For this review, take the finished solid that the model builds, in its own axes (mm). A direction names the side the tool comes from. Coordinates: 2 decimals unless noted, no trailing zeros. Write each loop counter-clockwise with the first axis right and the second up, starting at its lowest first coordinate (ties: lowest second). Pieces come first, ordered by that corner, then holes. Notation, with made-up numbers: M 4,16 L 63,16 A18 cw 63,31 Z; hole C 81,-31.75 d7. An arc over 180 degrees is marked long. Return JSON: item names as keys, results as strings.
```python
from build123d import *

# Parameters (mm, degrees)
F0_R     = 12.7
F1_DEPTH = 25.4
F2_R     = 6.35
F3_DEPTH = 12.7
F4_R     = 9.525
F5_DEPTH = 50.8


with BuildPart() as f1:
    # F0 (on Front) → F1 (new body)
    with BuildSketch(Plane.XZ):
        Circle(F0_R)
    extrude(amount=F1_DEPTH)

    # F2 (on face) → F3 (join)
    with BuildSketch(Plane(origin=(0, 0, 0), x_dir=(-1, 0, 0), z_dir=(0, 1, 0))):
        Circle(F2_R)
    extrude(amount=F3_DEPTH)

    # F4 (on face) → F5 (join)
    with BuildSketch(Plane.XZ.offset(25.4)):
        Circle(F4_R)
    extrude(amount=F5_DEPTH)


solid = f1.part
```
1. We need section D-D (y = -29). State the section outline as (x, z) points (3 decimals), plus the area to 3 significant figures.
Checks:
{"outline": "C 0,0 d19.05", "area": "285 mm2"}
2. Clearance check with flat-ended pins moving along their axes: pin 1 Ø6 at (x, y) = (4, -15) entering from +Z; pin 2 Ø6 at (x, y) = (6.5, -30) entering from -Z; pin 3 Ø4 at (x, z) = (-5, 8.5) entering from +Y. State where each tip first meets the part, or that it passes through.
Checks:
{"pin 1": "z = 12.66", "pin 2": "z = -8.86", "pin 3": "y = 0"}
3. Wall thickness on L1, parallel to Y at x = -9, z = 1.25; L2, parallel to Z at x = 0, y = -6; L3, parallel to Y at x = 3, z = -10.75: over which ranges is each line inside the solid? List them lowest first. Write a range as from..to.
Checks:
{"L1": "-76.2..0", "L2": "-12.7..12.7", "L3": "-25.4..0"}
4. We need section C-C (y = 1.5). State the section outline as (x, z) points, plus the area to 3 significant figures.
Checks:
{"outline": "C 0,0 d12.7", "area": "127 mm2"}
5. We need section A-A (x = 0). State the section outline as (y, z) points (3 decimals), plus the area to 3 significant figures.
Checks:
{"outline": "M -76.2,-9.525 L -25.4,-9.525 L -25.4,-12.7 L 0,-12.7 L 0,-6.35 L 12.7,-6.35 L 12.7,6.35 L 0,6.35 L 0,12.7 L -25.4,12.7 L -25.4,9.525 L -76.2,9.525 Z", "area": "1,770 mm2"}
6. For faces 1 (the face through (-2.75, -12.52, -12.4)), 2 (the face through (3, 0, 6)), 3 (the face through (5, -25.4, 9)), list the 3-axis set-ups (+Z, -Z, +X, -X, +Y, -Y) from which the entire face can be reached by the end or side of a thin tool; tool diameter is ignored.
Checks:
{"face 1": "+Y, -Y", "face 2": "+Y", "face 3": "-Y"}
7. We need section B-B (z = 0). State the section outline as (x, y) points (3 decimals).
Checks:
{"outline": "M -12.7,-25.4 L -9.525,-25.4 L -9.525,-76.2 L 9.525,-76.2 L 9.525,-25.4 L 12.7,-25.4 L 12.7,0 L 6.35,0 L 6.35,12.7 L -6.35,12.7 L -6.35,0 L -12.7,0 Z"}
